```python
from build123d import *

# Parameters (mm, degrees)
BOSS_EXTRUDE1_DEPTH = 200
REVOLVE1_ANGLE      = 90
SKETCH7_W           = 11.8
SKETCH7_H           = 29.9
CUT_EXTRUDE1_DEPTH  = 22.5
CUT_EXTRUDE2_START  = 17.4
CUT_EXTRUDE2_DEPTH  = 15
CUT_EXTRUDE3_START  = -22.5
SKETCH7_4_W         = 11.8
SKETCH7_4_H         = 2.7
CUT_EXTRUDE3_DEPTH  = 4.7
LPATTERN1_COUNT     = 2
LPATTERN1_PITCH     = 80
CUT_EXTRUDE4_START  = -45
SKETCH9_W           = 12
SKETCH9_H           = 31.9
CUT_EXTRUDE4_DEPTH  = 15
CUT_EXTRUDE5_START  = -30
SKETCH9_3_W         = 12
SKETCH9_3_H         = 22.5
CUT_EXTRUDE5_DEPTH  = 15.9
CUT_EXTRUDE7_START  = -30
SKETCH9_4_R         = 0.5
CUT_EXTRUDE7_DEPTH  = 1


# Read off the part's stored shape, not the designer's step: Cut-Extrude2
with BuildPart() as part:
    # Sketch1 → Boss-Extrude1 (new body)
    with BuildSketch(Plane.XY):
        with BuildLine():
            Line((-37.5, 45), (37.5, 45))
            add(Edge.make_bspline(
                [(-37.5, 45), (-36.538066416, -13.829055166), (35.114143496, -16.15963011), (37.5, 45)],
                knots=[0, 0, 0, 0, 1, 1, 1, 1], degree=3))
        make_face()
    extrude(amount=BOSS_EXTRUDE1_DEPTH)

    # Sketch1<2> → Revolve1 (revolve)
    with BuildSketch(Plane.XY):
        with BuildLine():
            Line((37.5, 45), (-37.5, 45))
            add(Edge.make_bspline(
                [(-37.5, 45), (-36.538066416, -13.829055166), (35.114143496, -16.15963011), (37.5, 45)],
                knots=[0, 0, 0, 0, 1, 1, 1, 1], degree=3))
        make_face()
    revolve(axis=Axis((-37.5, 45, 0), (1, 0, 0)), revolution_arc=REVOLVE1_ANGLE)

    # Sketch7 → Cut-Extrude1 (cut)
    with BuildSketch(Plane(origin=(0, 45, 0), x_dir=(1, 0, 0), z_dir=(0, 1, 0))):
        with Locations((-17.5, -2.45)):
            Rectangle(SKETCH7_W, SKETCH7_H)
        with Locations((17.5, -2.45)):
            Rectangle(SKETCH7_W, SKETCH7_H)
        with Locations((-17.5, -47.35)):
            Rectangle(SKETCH7_W, SKETCH7_H)
        with Locations((17.5, -47.35)):
            Rectangle(SKETCH7_W, SKETCH7_H)
    cut_extrude1 = extrude(amount=-CUT_EXTRUDE1_DEPTH, mode=Mode.SUBTRACT)

    # Cut-Extrude2 outline → Cut-Extrude2 (cut)
    with BuildSketch(Plane.XY.offset(CUT_EXTRUDE2_START)):
        with BuildLine():
            Line((35.498438873, 45), (-35.499725066, 45))
            add(Edge.make_bspline(
                [(-35.499725066, 45), (-35.368650609, 37.205082169), (-34.301979481, 30.199561306), (-32.413613618, 23.984635954), (-29.817810175, 18.556811549), (-26.625334767, 13.909452625), (-22.944999564, 10.026846468), (-18.86488359, 6.899280201), (-14.482583961, 4.530449937), (-9.895330776, 2.922239991), (-5.202441131, 2.078686183), (4.195747969, 1.92933157), (8.901042205, 2.622767579), (13.515468258, 4.088792702), (17.941749121, 6.331594499), (22.084774291, 9.360328131), (25.852428778, 13.179838208), (29.158791013, 17.820930982), (31.88915848, 23.308583975), (33.93262988, 29.659944885), (35.173667519, 36.887661716), (35.498438873, 45)],
                knots=[0.000190564, 0.000190564, 0.000190564, 0.000190564, 0.000190564, 0.000190564, 0.000190564, 0.000190564, 0.000190564, 0.000190564, 0.000190564, 0.000190564, 0.5, 0.5, 0.5, 0.5, 0.5, 0.5, 0.5, 0.5, 0.5, 0.5, 0.999563761, 0.999563761, 0.999563761, 0.999563761, 0.999563761, 0.999563761, 0.999563761, 0.999563761, 0.999563761, 0.999563761, 0.999563761, 0.999563761], degree=11))
        make_face()
    cut_extrude2 = extrude(amount=CUT_EXTRUDE2_DEPTH, mode=Mode.SUBTRACT)

    # Sketch7<4> → Cut-Extrude3 (cut)
    with BuildSketch(Plane(origin=(0, 45, 0), x_dir=(1, 0, 0), z_dir=(0, 1, 0)).offset(CUT_EXTRUDE3_START)):
        with Locations((-17.5, -4.65)):
            Rectangle(SKETCH7_4_W, SKETCH7_4_H)
        with Locations((17.5, -4.55)):
            Rectangle(SKETCH7_4_W, SKETCH7_4_H)
        with Locations((17.5, -45.15)):
            Rectangle(SKETCH7_4_W, SKETCH7_4_H)
        with Locations((-17.5, -45.15)):
            Rectangle(SKETCH7_4_W, SKETCH7_4_H)
    cut_extrude3 = extrude(amount=-CUT_EXTRUDE3_DEPTH, mode=Mode.SUBTRACT)

    # LPattern1: Cut-Extrude1, Cut-Extrude2, Cut-Extrude3 ×2
    with Locations(*[(0, 0, i * LPATTERN1_PITCH) for i in range(1, LPATTERN1_COUNT)]):
        add(cut_extrude1, mode=Mode.SUBTRACT)
        add(cut_extrude2, mode=Mode.SUBTRACT)
        add(cut_extrude3, mode=Mode.SUBTRACT)

    # Sketch9 → Cut-Extrude4 (cut)
    with BuildSketch(Plane(origin=(0, 45, 0), x_dir=(1, 0, 0), z_dir=(0, 1, 0)).offset(CUT_EXTRUDE4_START)):
        with Locations((0, -184.05)):
            Rectangle(SKETCH9_W, SKETCH9_H)
    extrude(amount=CUT_EXTRUDE4_DEPTH, mode=Mode.SUBTRACT)

    # Sketch9<3> → Cut-Extrude5 (cut)
    with BuildSketch(Plane(origin=(0, 45, 0), x_dir=(1, 0, 0), z_dir=(0, 1, 0)).offset(CUT_EXTRUDE5_START)):
        with Locations((0, -184.05)):
            Rectangle(SKETCH9_3_W, SKETCH9_3_H)
    extrude(amount=CUT_EXTRUDE5_DEPTH, mode=Mode.SUBTRACT)

    # Sketch9<4> → Cut-Extrude7 (cut)
    with BuildSketch(Plane(origin=(0, 45, 0), x_dir=(1, 0, 0), z_dir=(0, 1, 0)).offset(CUT_EXTRUDE7_START)):
        with Locations(Location((0, -170.4, 0), (0, 0, 270))):
            Circle(SKETCH9_4_R)
        with Locations(Location((0, -197.7, 0), (0, 0, 270))):
            Circle(SKETCH9_4_R)
    extrude(amount=CUT_EXTRUDE7_DEPTH, mode=Mode.SUBTRACT)


solid = part.part
```
Model file for the job. Use its own axes, mm. A direction names the side the tool comes from. Give positions to 0.01 mm unless a question says otherwise; leave off trailing zeros. One line per item, written item: value. Start each with the question number.
1. Probe L1, parallel to X at y = 31, z = 49; L2, parallel to Z at x = -27.5, y = 22; L3, parallel to Z at x = 13.5, y = 33. List the from-to ranges inside material, lowest first. Write a range as from..to.
2. Pull direction Z, two halves, no side cores. Call faces 3 (the flat face through (17, 20, 85.9)), 4 (the flat face through (0, 7, 168.1)): pulls with the +Z half, pulls with the -Z half, needs draft (parallel to the pull), parting line crosses it, or undercut.
3. Slice it at A-A (y = 20). Give the number of separate pieces and of enclosed holes in the cut face, plus the area to 3 significant figures.
4. Pin check, flat tips, straight feed: pin 1 (2 mm diameter, centred on y = 32, z = -15, fed in from -X); pin 2 (5.5 mm diameter, centred on x = 17.5, z = 118, fed in from +Y); pin 3 (5 mm diameter, centred on x = 16, y = 19.5, fed in from -Z); pin 4 (13 mm diameter, centred on x = -18, z = 72, fed in from +Y). Stop position of each tip, or through.
5. Which spindle directions (+Z, -Z, +X, -X, +Y, -Y) get a long thin tool onto all of the face, cutting with end or side? Do faces 1 (the flat face through (0, 30.9, 184)), 2 (the flat face through (11.6, 32, 48)). Say none if no direction does.
Solution:
1. L1: x = -35.75..-23.4, -11.6..11.6, 23.4..35.53
1. L2: z = -21.25..17.4, 32.4..97.4, 112.4..200
1. L3: z = -40.42..-12.5, 62.3..67.5, 142.3..200
2. face 3: undercut
2. face 4: pulls with the +Z half
3. separate pieces: 1
3. enclosed holes: 11
3. area: 12,200 mm^2
4. pin 1: stops at x = -34.3
4. pin 2: stops at y = 22.5
4. pin 3: stops at z = -34.46
4. pin 4: stops at y = 45
5. face 1: -Y
5. face 2: +Y
